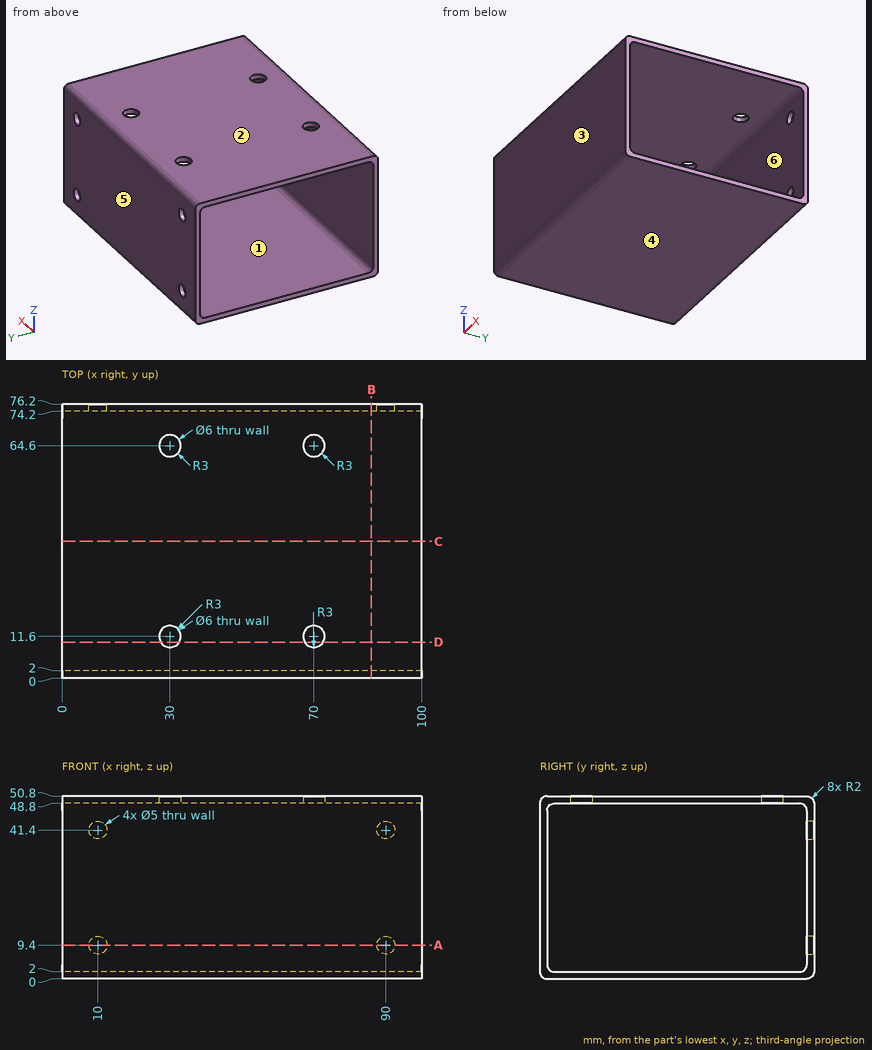
Could you check a few things on this drawing? It's one solid part, dimensions in mm from its lowest x, y, z. A direction names the side the tool comes from. Round coordinates to 2 decimals unless told otherwise and drop trailing zeros. Loops run counter-clockwise (first coordinate to the right, second up) from the corner with the lowest first, then second, coordinate; pieces in that order, holes last. Notation, with made-up numbers: (75.5, -6) -> (100.5, -6) arc R14 cw to (100.5, 17) -> close; hole circle Ø9 at (-16, 12.5). An arc over 180 degrees is marked (long way). One line per item, written item: value. Start each with the question number.
1. If we section it at A-A, the plane z = 9.4: Write out the boundary of the cut face in (x, y), then the cut area to 3 significant figures.
2. If we mould it in two halves opening along Z, with no side actions, what happens to the marked faces 1, 2, 3 and 4? For each: pulls with the +Z half, pulls with the -Z half, needs draft (parallel to the pull), parting line crosses it, or undercut.
3. For the marked faces 5 and 6, which set-ups out of +Z, -Z, +X, -X, +Y, -Y let a thin tool reach every point of the face, with its end or its side?
4. If we section it at C-C, the plane y = 38: Write out the boundary of the cut face in (x, z), then the cut area to 3 significant figures.
5. If I drill on probe 1 along X at (y, z) = (74.9, 41.4); probe 2 along Y at (x, z) = (82.5, 44); probe 3 along Z at (x, y) = (18, 6), over which ranges is the centre line in solid material (lowest first)?
6. If we section it at B-B, the plane x = 86: Write out the boundary of the cut face in (y, z).
7. If we section it at D-D, the plane y = 10: Write out the boundary of the cut face in (x, z).
8. For pin 1 (5 mm diameter, centred on x = 30, y = 64.6, fed in from +Z); pin 2 (4.5 mm diameter, centred on x = 90, z = 9.4, fed in from +Y), each with a flat end and sliding along its axis, tell me the tip position at first contact or that it passes through.
Calculated:
1. outline: (0, 0) -> (100, 0) -> (100, 2) -> (0, 2) -> close; (0, 74.2) -> (7.5, 74.2) -> (7.5, 76.2) -> (0, 76.2) -> close; (12.5, 74.2) -> (87.5, 74.2) -> (87.5, 76.2) -> (12.5, 76.2) -> close; (92.5, 74.2) -> (100, 74.2) -> (100, 76.2) -> (92.5, 76.2) -> close
1. area: 380 mm²
2. face 1: undercut
2. face 2: pulls with the +Z half
2. face 3: needs draft
2. face 4: pulls with the -Z half
3. face 5: +Z, -Z, +X, -X, +Y
3. face 6: +X, -X
4. outline: (0, 0) -> (100, 0) -> (100, 2) -> (0, 2) -> close; (0, 48.8) -> (100, 48.8) -> (100, 50.8) -> (0, 50.8) -> close
4. area: 400 mm²
5. probe 1: x = 0 to 7.5, 12.5 to 87.5, 92.5 to 100
5. probe 2: y = 0 to 2, 74.2 to 76.2
5. probe 3: z = 0 to 2, 48.8 to 50.8
6. outline: (0, 2) arc R2 ccw to (2, 0) -> (74.2, 0) arc R2 ccw to (76.2, 2) -> (76.2, 48.8) arc R2 ccw to (74.2, 50.8) -> (2, 50.8) arc R2 ccw to (0, 48.8) -> close; hole (2, 4) arc R2 ccw to (4, 2) -> (72.2, 2) arc R2 ccw to (74.2, 4) -> (74.2, 46.8) arc R2 ccw to (72.2, 48.8) -> (4, 48.8) arc R2 ccw to (2, 46.8) -> close
7. outline: (0, 0) -> (100, 0) -> (100, 2) -> (0, 2) -> close; (0, 48.8) -> (27.46, 48.8) -> (27.46, 50.8) -> (0, 50.8) -> close; (32.54, 48.8) -> (67.46, 48.8) -> (67.46, 50.8) -> (32.54, 50.8) -> close; (72.54, 48.8) -> (100, 48.8) -> (100, 50.8) -> (72.54, 50.8) -> close
8. pin 1: stops at z = 2
8. pin 2: stops at y = 2
